```python
from build123d import *

# Parameters (mm, degrees)
SKETCH_1_R          = 9.5
EXTRUDE_1_DEPTH     = 10
SKETCH_2_W          = 20
SKETCH_2_H          = 30
EXTRUDE_2_DEPTH     = 210
SKETCH_3_W          = 20
SKETCH_3_H          = 30
EXTRUDE_3_DEPTH     = 70
EXTRUDE_4_DEPTH     = 20
SKETCH_5_R          = 3
CUT_EXTRUDE_1_DEPTH = 20


with BuildPart() as part:
    # Sketch 1 → Extrude 1 (new body)
    with BuildSketch(Plane.XY):
        with BuildLine():
            Line((0, 15), (100, 15))
            Line((100, 15), (100, -15))
            Line((100, -15), (0, -15))
            ThreePointArc((0, -15), (-15, 0), (0, 15))
        make_face()
        Circle(SKETCH_1_R, mode=Mode.SUBTRACT)
    extrude(amount=EXTRUDE_1_DEPTH)

    # Sketch 2 → Extrude 2 (add)
    with BuildSketch(Plane(origin=(0, 0, 0), x_dir=(-1, 0, 0), z_dir=(0, 0, -1))):
        with Locations((-90, 0)):
            Rectangle(SKETCH_2_W, SKETCH_2_H)
    extrude(amount=EXTRUDE_2_DEPTH)

    # Sketch 3 → Extrude 3 (add)
    with BuildSketch(Plane.ZY.offset(-80)):
        with Locations((-200, 0)):
            Rectangle(SKETCH_3_W, SKETCH_3_H)
    extrude(amount=EXTRUDE_3_DEPTH)

    # Sketch 4 → Extrude 4 (add)
    with BuildSketch(Plane.ZY.offset(-10)):
        Polygon((-190, 0), (-190, -220), (30, -220), (30, -240), (-210, -240), (-210, 0), align=None)
    extrude_4 = extrude(amount=EXTRUDE_4_DEPTH)

    # Mirror 1: Extrude 4 across plane
    add(extrude_4.mirror(Plane(origin=(-10, 0, -210), x_dir=(0, 0, 1), z_dir=(0, -1, 0))))

    # Sketch 5 → Cut-Extrude 1 (cut)
    with BuildSketch(Plane(origin=(0, -220, 0), x_dir=(1, 0, 0), z_dir=(0, 1, 0))):
        with Locations(Location((0, -5, 0), (0, 0, 270))):
            Circle(SKETCH_5_R)
    cut_extrude_1 = extrude(amount=-CUT_EXTRUDE_1_DEPTH, mode=Mode.SUBTRACT)

    # Mirror 2: Cut-Extrude 1 across plane
    add(cut_extrude_1.mirror(Plane.ZX), mode=Mode.SUBTRACT)


solid = part.part
```
Here's how the part is built. I have some questions about the finished solid (model axes, mm). A direction names the side the tool comes from. Coordinates: 2 decimals unless noted, no trailing zeros. Loops run counter-clockwise (first coordinate to the right, second up) from the corner with the lowest first, then second, coordinate; pieces in that order, holes last. Notation, with made-up numbers: (69, 63.25) - (103, 63.25) arc R19 cw to (103, 71.25) - close; hole circle Ø6 at (8.25, -31.75). An arc over 180 degrees is marked (long way). Answer as CSV lines item,"result".
Q1. If we section it at C-C, the plane z = -5: Write out the boundary of the cut face in (x, y), and give its area (3 significant figures).
Response:
outline,"(-10, -240) - (10, -240) - (10, -220) - (-10, -220) - close; (-10, 220) - (10, 220) - (10, 240) - (-10, 240) - close; (80, -15) - (100, -15) - (100, 15) - (80, 15) - close"
area,"1,400 mm2"
Q2. If we section it at A-A, the plane x = 43.5: Write out the boundary of the cut face in (y, z), and give its area (3 significant figures).
Response:
outline,"(-15, -210) - (15, -210) - (15, -190) - (-15, -190) - close; (-15, 0) - (15, 0) - (15, 10) - (-15, 10) - close"
area,"900 mm2"
Q3. For faces 4 (the face through (0, 220, -82)), 5 (the face through (10, -227, -143)), 6 (the face through (4.38, -8.43, 4.93)), which set-ups out of +Z, -Z, +X, -X, +Y, -Y let a thin tool reach every point of the face, with its end or its side?
Response:
face 4,"+Z, +X, -X"
face 5,"+Z, -Z, +X, -Y"
face 6,"+Z"
Q4. If I drill on L1, parallel to X at y = 227, z = 5; L2, parallel to Y at x = 5.5, z = -172; L3, parallel to Y at x = 0, z = 7.5, over which ranges is the centre line in solid material (lowest first)? Write a range as [from, to].
Response:
L1,"[-10, -3], [3, 10]"
L2,"[-240, -220], [220, 240]"
L3,"[-15, -9.5], [9.5, 15]"
Q5. If we section it at B-B, the plane y = 0: Write out the boundary of the cut face in (x, z), and give its area (3 significant figures).
Response:
outline,"(-15, 0) - (-9.5, 0) - (-9.5, 10) - (-15, 10) - close; (-10, -210) - (100, -210) - (100, 10) - (9.5, 10) - (9.5, 0) - (80, 0) - (80, -190) - (-10, -190) - close"
area,"6,960 mm2"
Q6. For pin 1 (24 mm diameter, centred on x = 66, y = -5.5, fed in from +Z); pin 2 (15 mm diameter, centred on y = -0.5, z = -92, fed in from -X); pin 3 (5.5 mm diameter, centred on x = 0, z = 5, fed in from -Y), each with a flat end and sliding along its axis, tell me the tip position at first contact or that it passes through.
Response:
pin 1,"z = 10"
pin 2,"x = 80"
pin 3,"y = -15"
Q7. We'd pull the mould along Z, two halves only. Please class faces 1 (the face through (33, 0, 0)), 2 (the face through (0, -240, -88)), 3 (the face through (0, 230, 30)): pulls with the +Z half, pulls with the -Z half, needs draft (parallel to the pull), parting line crosses it, or undercut.
Response:
face 1,"undercut"
face 2,"needs draft"
face 3,"pulls with the +Z half"
